Part model, mm, in its own coordinate system. Give positions to 0.01 mm unless a question says otherwise; leave off trailing zeros. Write each loop counter-clockwise with the first axis right and the second up, starting at its lowest first coordinate (ties: lowest second). Pieces come first, ordered by that corner, then holes. Notation, with made-up numbers: (86, 0) - (100, 0) arc R19 ccw to (100, 8) - close; hole circle Ø1 at (41.25, 35). An arc over 180 degrees is marked (long way). Answer in a Markdown table with one row per item. Add a question column.
1. Pull direction Y, two halves, no side cores. Call faces 1 (the flat face through (-14, 0, -7)), 2 (the cylindrical face through (-16.45, 148.226, -0.923)), 3 (the flat face through (-14, 162, -7)): released by +Y, released by -Y, zero draft, split by the parting line, or undercut.
2. Probe line 1 along Y through (x, z) = (-16, 0); line 2 along Z through (x, y) = (-1, 36); line 3 along Z through (x, y) = (-5.5, 79). List the from-to ranges inside material, lowest first.
3. Drop flat-ended pins along their axis: pin 1 Ø1 at (x, y) = (2.5, 73) entering from +Z; pin 2 Ø1.5 at (y, z) = (117, 5.5) entering from +X; pin 3 Ø3 at (x, y) = (6, 66.5) entering from -Z. Give the stop position or say it passes through.
4. Band-saw the part on A-A on x = 0. Write the cut outline in (y, z), plus the area to 3 significant figures.
```python
from build123d import *

# Parameters (mm, degrees)
ESQUISSE1_R                  = 17.5
ESQUISSE1_R_2                = 15.5
BOSS_EXTRU_1_DEPTH           = 162
ENL_V_MAT_EXTRU_1_DEPTH      = 164.879528923
ENL_V_MAT_EXTRU_1_DEPTH_BACK = 164.879528923
ESQUISSE2_R                  = 2


with BuildPart() as part:
    # Esquisse1 → Boss.-Extru.1 (new body)
    with BuildSketch(Plane(origin=(0, 0, 0), x_dir=(1, 0, 0), z_dir=(0, 1, 0))):
        with Locations(Location((0, 0, 0), (0, 0, 270))):
            Circle(ESQUISSE1_R)
        with Locations(Location((0, 0, 0), (0, 0, 270))):
            Circle(ESQUISSE1_R_2, mode=Mode.SUBTRACT)
    extrude(amount=BOSS_EXTRU_1_DEPTH)

    # Esquisse2 → Enlèv. mat.-Extru.1 (cut, two sides: drawn at the far end of the back side and taken through both)
    with BuildSketch(Plane(origin=(0, 0, 0), x_dir=(0, 0, -1), z_dir=(1, 0, 0)).offset(-ENL_V_MAT_EXTRU_1_DEPTH_BACK)):
        with Locations((0, 150)):
            Circle(ESQUISSE2_R)
        with Locations((0, 12)):
            Circle(ESQUISSE2_R)
    extrude(amount=ENL_V_MAT_EXTRU_1_DEPTH + ENL_V_MAT_EXTRU_1_DEPTH_BACK, mode=Mode.SUBTRACT)


solid = part.part
```
Values:
| question | item | result |
|---|---|---|
| 1 | face 1 | released by -Y |
| 1 | face 2 | undercut |
| 1 | face 3 | released by +Y |
| 2 | line 1 | y = 0 to 10, 14 to 148, 152 to 162 |
| 2 | line 2 | z = -17.47 to -15.47, 15.47 to 17.47 |
| 2 | line 3 | z = -16.61 to -14.49, 14.49 to 16.61 |
| 3 | pin 1 | stops at z = 17.39 |
| 3 | pin 2 | stops at x = 16.84 |
| 3 | pin 3 | stops at z = -16.91 |
| 4 | outline | (0, -17.5) - (162, -17.5) - (162, -15.5) - (0, -15.5) - close; (0, 15.5) - (162, 15.5) - (162, 17.5) - (0, 17.5) - close |
| 4 | area | 648 mm² |
